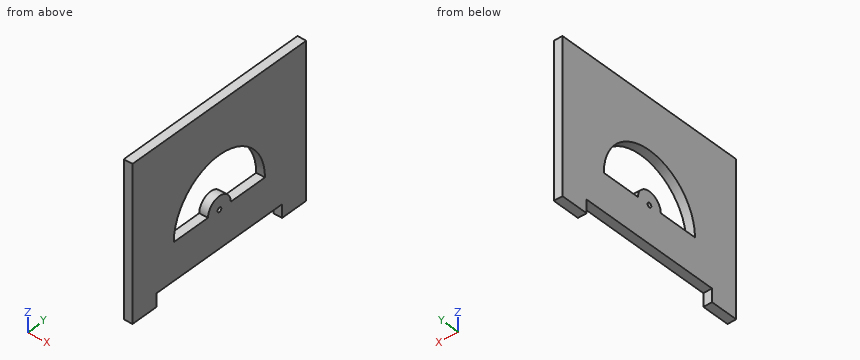
```python
from build123d import *

# Parameters (mm, degrees)
F0_W     = 228.6
F0_H     = 175
F1_DEPTH = 10
F7_DEPTH = 25
F3_W     = 165
F3_H     = 30
F4_DEPTH = 25
F9_D     = 5


with BuildPart() as f1:
    # F0 (on Right) → F1 (new body)
    with BuildSketch(Plane.YZ):
        Rectangle(F0_W, F0_H)
    extrude(amount=F1_DEPTH)

    # F2 (on face) → F7 (cut)
    with BuildSketch(Plane.YZ.offset(10)):
        with BuildLine():
            Line((15, -30), (60, -30))
            ThreePointArc((60, -30), (0, 30), (-60, -30))
            Line((-60, -30), (-15, -30))
            ThreePointArc((-15, -30), (0, -15), (15, -30))
        make_face()
    extrude(amount=-F7_DEPTH, mode=Mode.SUBTRACT)

    # F3 (on face) → F4 (cut)
    with BuildSketch(Plane.YZ.offset(10)):
        with Locations((0, -87.5)):
            Rectangle(F3_W, F3_H)
    extrude(amount=-F4_DEPTH, mode=Mode.SUBTRACT)

    # F9 (through all)
    with Locations(Plane.YZ.offset(10)):
        with Locations((0, -30)):
            Hole(F9_D / 2)


solid = f1.part
```
CAD build for the part. Positions are in the model's coordinates, mm. Coordinates: 2 decimals unless noted, no trailing zeros. Order: outer loops, then holes, each group sorted by start corner. A loop starts at its lowest first (then second) coordinate and runs counter-clockwise, first axis right, second up. Notation, with made-up numbers: (85, 72) - (113, 72) arc R19 ccw to (113, 88) - close; hole circle Ø4 at (-29.75, 23). An arc over 180 degrees is marked (long way). Use a Markdown table: item, result. Add a question column.
(1) Saw through at D-D (z = 1.5). Give the cut face in (x, y), then the cut area to 3 significant figures.
(2) Saw through at A-A (y = 0). Give the cut face in (x, z).
(3) Saw through at C-C (y = 50). Give the cut face in (x, z), then the cut area to 3 significant figures.
(4) Saw through at B-B (x = 2). Give the cut face in (y, z), then the cut area to 3 significant figures.
(5) Drill centre lines: line 1 along Z through (x, y) = (5.25, 0); line 2 along Z through (x, y) = (2.75, -10); line 3 along Y through (x, z) = (7.75, -11). Where is each one in solid material? Low to high. Write a range as [from, to].
Solved:
| question | item | result |
|---|---|---|
| 1 | outline | (0, -114.3) - (10, -114.3) - (10, -51.07) - (0, -51.07) - close; (0, 51.07) - (10, 51.07) - (10, 114.3) - (0, 114.3) - close |
| 1 | area | 1,260 mm² |
| 2 | outline | (0, -72.5) - (10, -72.5) - (10, -32.5) - (0, -32.5) - close; (0, -27.5) - (10, -27.5) - (10, -15) - (0, -15) - close; (0, 30) - (10, 30) - (10, 87.5) - (0, 87.5) - close |
| 3 | outline | (0, -72.5) - (10, -72.5) - (10, -30) - (0, -30) - close; (0, 3.17) - (10, 3.17) - (10, 87.5) - (0, 87.5) - close |
| 3 | area | 1,270 mm² |
| 4 | outline | (-114.3, -87.5) - (-82.5, -87.5) - (-82.5, -72.5) - (82.5, -72.5) - (82.5, -87.5) - (114.3, -87.5) - (114.3, 87.5) - (-114.3, 87.5) - close; hole (-60, -30) - (-15, -30) arc R15 cw to (15, -30) - (60, -30) arc R60 ccw to start; hole circle Ø5 at (0, -30) |
| 4 | area | 32,200 mm² |
| 5 | line 1 | z = [-72.5, -32.5], [-27.5, -15], [30, 87.5] |
| 5 | line 2 | z = [-72.5, -18.82], [29.16, 87.5] |
| 5 | line 3 | y = [-114.3, -56.91], [56.91, 114.3] |
